```python
from build123d import *

# Parameters (mm, degrees)
SKETCH1_W           = 129.7
SKETCH1_H           = 180
SKETCH1_R           = 2.5
SKETCH1_R_2         = 3.6
BOSS_EXTRUDE1_DEPTH = 5
FILLET1_R           = 3


with BuildPart() as part:
    # Sketch1 → Boss-Extrude1 (new body)
    with BuildSketch(Plane.XY):
        with Locations((64.85, 90)):
            Rectangle(SKETCH1_W, SKETCH1_H)
        with Locations((15, 15)):
            Circle(SKETCH1_R, mode=Mode.SUBTRACT)
        with Locations((15, 165)):
            Circle(SKETCH1_R, mode=Mode.SUBTRACT)
        with Locations((114.7, 165)):
            Circle(SKETCH1_R_2, mode=Mode.SUBTRACT)
        with Locations((114.7, 15)):
            Circle(SKETCH1_R_2, mode=Mode.SUBTRACT)
        with Locations((34.85, 160)):
            Circle(SKETCH1_R, mode=Mode.SUBTRACT)
        with Locations((64.85, 160)):
            Circle(SKETCH1_R, mode=Mode.SUBTRACT)
        with Locations((94.85, 160)):
            Circle(SKETCH1_R, mode=Mode.SUBTRACT)
        with Locations((34.85, 60)):
            Circle(SKETCH1_R, mode=Mode.SUBTRACT)
        with Locations((64.85, 60)):
            Circle(SKETCH1_R, mode=Mode.SUBTRACT)
        with Locations((94.85, 60)):
            Circle(SKETCH1_R, mode=Mode.SUBTRACT)
    extrude(amount=BOSS_EXTRUDE1_DEPTH)

    # Fillet1
    fillet1_edges = [part.edges().sort_by_distance(p)[0] for p in [
        (0, 180, 2.5),
        (129.7, 180, 2.5),
        (129.7, 0, 2.5),
        (0, 0, 2.5),
    ]]
    fillet(fillet1_edges, radius=FILLET1_R)


solid = part.part
```
CAD build for the part. Positions are in the model's coordinates, mm. Coordinates: 2 decimals unless noted, no trailing zeros. Order: outer loops, then holes, each group sorted by start corner. A loop starts at its lowest first (then second) coordinate and runs counter-clockwise, first axis right, second up. Notation, with made-up numbers: (-13, -13.5) -> (-5, -13.5) arc R7 ccw to (-5, -1.5) -> close; hole circle Ø10 at (13.25, -5). An arc over 180 degrees is marked (long way). Use one line per item in the form item = value. Start each with the question number.
1) Band-saw the part on B-B on y = 165. Give the cut face in (x, z), then the cut area to 4 significant figures.
2) Drill centre lines: L1, parallel to Y at x = 34.85, z = 4; L2, parallel to Y at x = 114.7, z = 1.3; L3, parallel to X at y = 165, z = 3.85. Where is each one in solid material? Low to high. Write a range as [from, to].
3) Pull direction Y, two halves, no side cores. Call faces 1 (the flat face through (64, 0, 2)), 2 (the cylindrical face through (66.19, 162.11, 2.46)), 3 (the flat face through (64, 91, 5)): +Y half, -Y half, draft (parallel to the pull), parting line (faces both ways), or undercut.
4) Band-saw the part on A-A on x = 64.85. Give the cut face in (y, z).
Entries:
q1.outline = (0, 0) -> (12.5, 0) -> (12.5, 5) -> (0, 5) -> close; (17.5, 0) -> (111.1, 0) -> (111.1, 5) -> (17.5, 5) -> close; (118.3, 0) -> (129.7, 0) -> (129.7, 5) -> (118.3, 5) -> close
q1.area = 587.5 mm2
q2.L1 = [0, 57.5], [62.5, 157.5], [162.5, 180]
q2.L2 = [0, 11.4], [18.6, 161.4], [168.6, 180]
q2.L3 = [0, 12.5], [17.5, 111.1], [118.3, 129.7]
q3.face_1 = -Y half
q3.face_2 = undercut
q3.face_3 = draft
q4.outline = (0, 0) -> (57.5, 0) -> (57.5, 5) -> (0, 5) -> close; (62.5, 0) -> (157.5, 0) -> (157.5, 5) -> (62.5, 5) -> close; (162.5, 0) -> (180, 0) -> (180, 5) -> (162.5, 5) -> close
